from build123d import *

# Parameters (mm, degrees)
F0_W     = 69
F0_H     = 27
F1_DEPTH = 2
F2_W     = 22
F2_H     = 22
F3_DEPTH = 8
F4_W     = 35
F4_H     = 18
F5_DEPTH = 5
F6_W     = 15
F6_H     = 12
F7_DEPTH = 5
F8_R     = 5.5
F9_DEPTH = 8.5


with BuildPart() as f1:
    # F0 (on Front) → F1 (new body)
    with BuildSketch(Plane.XZ):
        Rectangle(F0_W, F0_H)
    extrude(amount=F1_DEPTH)

    # F2 (on face) → F3 (join)
    with BuildSketch(Plane.XZ.offset(2)):
        with Locations((-31, 0)):
            Rectangle(F2_W, F2_H)
    extrude(amount=F3_DEPTH)

    # F4 (on face) → F5 (join)
    with BuildSketch(Plane.XZ.offset(2)):
        Rectangle(F4_W, F4_H)
    extrude(amount=F5_DEPTH)

    # F6 (on face) → F7 (join)
    with BuildSketch(Plane.XZ.offset(2)):
        with Locations((25, 5.5)):
            Rectangle(F6_W, F6_H)
    extrude(amount=F7_DEPTH)

    # F8 (on face) → F9 (join)
    with BuildSketch(Plane.XZ.offset(2)):
        with Locations((26.5, -8)):
            Circle(F8_R)
    extrude(amount=F9_DEPTH)


solid = f1.part
Could you check a few things on this model? Use its own coordinates, in mm. A direction names the side the tool comes from. Round coordinates to 2 decimals unless told otherwise and drop trailing zeros. Order: outer loops, then holes, each group sorted by start corner. A loop starts at its lowest first (then second) coordinate and runs counter-clockwise, first axis right, second up.
(1) I'm going to push flat-ended pins straight in: pin 1 (3 mm diameter, centred on y = -4.5, z = -6.5, fed in from +X); pin 2 (8 mm diameter, centred on x = -5, z = 8, fed in from -Y); pin 3 (5 mm diameter, centred on x = -20, y = -8.5, fed in from +Z). Where does each tip first touch, or does it pass through?
Response values:
pin 1: stops at x = 32
pin 2: stops at y = -7
pin 3: stops at z = 11
(2) Imagine slicing it at C-C (x = -14.5). Write out the boundary of the cut face in (y, z), plus the area to 3 significant figures.
Response values:
outline: (-7, -9) - (-2, -9) - (-2, -13.5) - (0, -13.5) - (0, 13.5) - (-2, 13.5) - (-2, 9) - (-7, 9) - close
area: 144 mm2
(3) Please list where these lines run through material, in increasing order: line 1 along X through (y, z) = (-2.75, 10.75); line 2 along X through (y, z) = (-4, -1.75); line 3 along X through (y, z) = (-1.25, 7.75).
Response values:
line 1: x = -42 to -20, 17.5 to 32.5
line 2: x = -42 to -20, -17.5 to 17.5
line 3: x = -34.5 to 34.5
(4) Imagine slicing it at A-A (y = -4.5). Write out the boundary of the cut face in (x, z).
Response values:
outline: (-42, -11) - (-20, -11) - (-20, 11) - (-42, 11) - close; (-17.5, -9) - (17.5, -9) - (17.5, -0.5) - (32.5, -0.5) - (32.5, 11.5) - (17.5, 11.5) - (17.5, 9) - (-17.5, 9) - close; circle Ø11 at (26.5, -8)
(5) Which directions (+Z, -Z, +X, -X, +Y, -Y) give clear straight access to the entire face, cutting with the end or side of a thin tool? Please do faces 1 (the flat face through (-31, -10, 0)), 2 (the flat face through (0, -4, 9)), 3 (the flat face through (25, -4, 11.5)), 4 (the flat face through (17.5, -4, -5)).
Response values:
face 1: +Z, -Z, -X, -Y
face 2: +Z, -Y
face 3: +Z, +X, -X, -Y
face 4: -Z, -Y
(6) Imagine slicing it at D-D (y = -8.75). Write out the boundary of the cut face in (x, z), plus the area to 3 significant figures.
Response values:
outline: (-42, -11) - (-20, -11) - (-20, 11) - (-42, 11) - close; circle Ø11 at (26.5, -8)
area: 579 mm2
(7) If we mould it in two halves opening along X, with no side actions, what happens to faces 5 (the flat face through (32.5, -4, 5)), 6 (the flat face through (-38, -2, 0)), 7 (the cylindrical face through (25.31, -6.19, -13.37)), 8 (the flat face through (7, -7, 1))? For each: released by +X, released by -X, zero draft, split by the parting line, or undercut.
Response values:
face 5: released by +X
face 6: zero draft
face 7: undercut
face 8: undercut
(8) Imagine slicing it at B-B (z = -8). Write out the boundary of the cut face in (x, y).
Response values:
outline: (-42, -10) - (-20, -10) - (-20, -2) - (-17.5, -2) - (-17.5, -7) - (17.5, -7) - (17.5, -2) - (21, -2) - (21, -10.5) - (32, -10.5) - (32, -2) - (34.5, -2) - (34.5, 0) - (-34.5, 0) - (-34.5, -2) - (-42, -2) - close
